For this review, use the dimensioned drawing (mm, ordinates from the lowest corner) and the shaded views. Coordinates: 2 decimals unless noted, no trailing zeros. Loops run counter-clockwise (first coordinate to the right, second up) from the corner with the lowest first, then second, coordinate; pieces in that order, holes last. Notation, with made-up numbers: (88, 54.25) - (134, 54.25) arc R6 cw to (134, 63.25) - close; hole circle Ø1 at (17.25, -30.5). An arc over 180 degrees is marked (long way). Use a Markdown table: item, result. Add a question column.
1) Add section B-B, the plane x = 40. Give the boundary of the cut face in (y, z).
2) Add section C-C, the plane y = 3.25. Give the boundary of the cut face in (x, z), and give its area (3 significant figures).
3) Clearance check with a flat-ended pin moving along its axis: pin 1 (1 mm diameter, centred on x = 60.5, z = 36, fed in from -Y). State where the tip first meets the part, or that it passes through.
4) The part is to be moulded in two halves that separate along X. For the marked faces 1, 2, 3 and 4, say which applies: pulls with the +X half, pulls with the -X half, needs draft (parallel to the pull), parting line crosses it, or undercut.
5) Add section A-A, the plane z = 20. Give the boundary of the cut face in (x, y), and give its area (3 significant figures).
6) To check wall thickness, follow L1, parallel to X at y = 3, z = 20; L2, parallel to X at y = 2.75, z = 3.5; L3, parallel to X at y = 5.25, z = 21. State the ranges of each line that lie inside material, in increasing order. Write a range as [from, to].
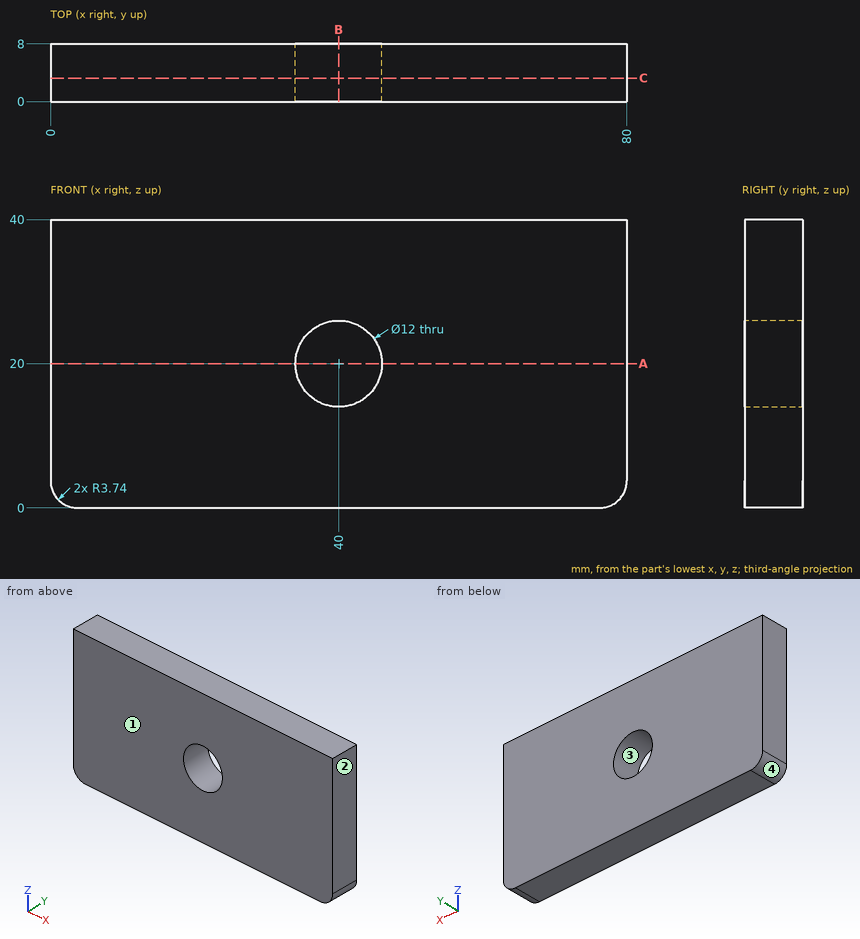
From the geometry:
| question | item | result |
|---|---|---|
| 1 | outline | (0, 0) - (8, 0) - (8, 14) - (0, 14) - close; (0, 26) - (8, 26) - (8, 40) - (0, 40) - close |
| 2 | outline | (0, 3.74) arc R3.74 ccw to (3.74, 0) - (76.26, 0) arc R3.74 ccw to (80, 3.74) - (80, 40) - (0, 40) - close; hole circle Ø12 at (40, 20) |
| 2 | area | 3,080 mm^2 |
| 3 | pin 1 | stops at y = 0 |
| 4 | face 1 | needs draft |
| 4 | face 2 | pulls with the +X half |
| 4 | face 3 | undercut |
| 4 | face 4 | pulls with the -X half |
| 5 | outline | (0, 0) - (34, 0) - (34, 8) - (0, 8) - close; (46, 0) - (80, 0) - (80, 8) - (46, 8) - close |
| 5 | area | 544 mm^2 |
| 6 | L1 | x = [0, 34], [46, 80] |
| 6 | L2 | x = [0.01, 79.99] |
| 6 | L3 | x = [0, 34.08], [45.92, 80] |
